```python
from build123d import *

# Parameters (mm, degrees)
BOSS_EXTRUDE1_DEPTH = 5.18
CUT_EXTRUDE4_REACH  = 45.046
SKETCH2_W           = 3.45
SKETCH2_H           = 5.15
CUT_EXTRUDE3_REACH  = 42.402
SKETCH7_R           = 1.575
SKETCH3_W           = 10.5
SKETCH3_H           = 30
SKETCH3_R           = 1.575
BOSS_EXTRUDE2_DEPTH = 1.5


with BuildPart() as part:
    # Sketch1 → Boss-Extrude1 (new body)
    with BuildSketch(Plane(origin=(0, 0, 0), x_dir=(0, 0, -1), z_dir=(1, 0, 0))):
        with BuildLine():
            Line((-5.5, -10.303333333), (-5.5, -17.953333333))
            Line((-5.5, -17.953333333), (3.25, -17.953333333))
            Line((3.25, -17.953333333), (3.25, -19.295))
            Line((3.25, -19.295), (1.25, -19.295))
            Line((1.25, -19.295), (1.25, -19.12))
            Line((1.25, -19.12), (-2.25, -19.12))
            Line((-2.25, -19.12), (-2.25, -19.295))
            Line((-2.25, -19.295), (-4.25, -19.295))
            Line((-4.25, -19.295), (-4.25, -19.12))
            Line((-4.25, -19.12), (-5.5, -19.12))
            Line((-5.5, -19.12), (-5.5, -23.37))
            Line((-5.5, -23.37), (-4.25, -23.37))
            Line((-4.25, -23.37), (-4.25, -23.195))
            Line((-4.25, -23.195), (-2.25, -23.195))
            Line((-2.25, -23.195), (-2.25, -23.37))
            Line((-2.25, -23.37), (1.25, -23.37))
            Line((1.25, -23.37), (1.25, -23.195))
            Line((1.25, -23.195), (3.25, -23.195))
            Line((3.25, -23.195), (3.25, -23.59))
            Line((3.25, -23.59), (-5.5, -23.59))
            Line((-5.5, -23.59), (-5.5, -28.59))
            Line((-5.5, -28.59), (5.72, -28.59))
            Line((5.72, -28.59), (5.72, -14.303333333))
            ThreePointArc((5.72, -14.303333333), (6.012893219, -13.596226552), (6.72, -13.303333333))
            Line((6.72, -13.303333333), (7.061666667, -13.303333333))
            Line((7.061666667, -13.303333333), (7.061666667, -15.303333333))
            Line((7.061666667, -15.303333333), (6.886666667, -15.303333333))
            Line((6.886666667, -15.303333333), (6.886666667, -25.34))
            Line((6.886666667, -25.34), (7.061666667, -25.34))
            Line((7.061666667, -25.34), (7.061666667, -27.34))
            Line((7.061666667, -27.34), (6.886666667, -27.34))
            Line((6.886666667, -27.34), (6.886666667, -28.59))
            Line((6.886666667, -28.59), (11.136666667, -28.59))
            Line((11.136666667, -28.59), (11.136666667, -27.34))
            Line((11.136666667, -27.34), (10.961666667, -27.34))
            Line((10.961666667, -27.34), (10.961666667, -25.34))
            Line((10.961666667, -25.34), (11.136666667, -25.34))
            Line((11.136666667, -25.34), (11.136666667, -15.303333333))
            Line((11.136666667, -15.303333333), (10.961666667, -15.303333333))
            Line((10.961666667, -15.303333333), (10.961666667, -13.303333333))
            Line((10.961666667, -13.303333333), (11.303333333, -13.303333333))
            ThreePointArc((11.303333333, -13.303333333), (12.010440115, -13.596226552), (12.303333333, -14.303333333))
            Line((12.303333333, -14.303333333), (12.303333333, -28.81))
            Line((12.303333333, -28.81), (-5.5, -28.81))
            Line((-5.5, -28.81), (-7, -30.31))
            Line((-7, -30.31), (-7, -36.14))
            Line((-7, -36.14), (-3, -36.14))
            Line((-3, -36.14), (-3, -34.64))
            Line((-3, -34.64), (-5.5, -34.64))
            Line((-5.5, -34.64), (-5.5, -31.31))
            Line((-5.5, -31.31), (17.303333333, -31.31))
            Line((17.303333333, -31.31), (13.803333333, -11.31))
            Line((13.803333333, -11.31), (13.803333333, 0))
            Line((13.803333333, 0), (0, 0))
            Line((0, 0), (0, -2))
            Line((0, -2), (12.303333333, -2))
            Line((12.303333333, -2), (12.303333333, -10.303333333))
            ThreePointArc((12.303333333, -10.303333333), (12.010440115, -11.010440115), (11.303333333, -11.303333333))
            Line((11.303333333, -11.303333333), (10.961666667, -11.303333333))
            Line((10.961666667, -11.303333333), (10.961666667, -9.303333333))
            Line((10.961666667, -9.303333333), (11.136666667, -9.303333333))
            Line((11.136666667, -9.303333333), (11.136666667, -5.47))
            Line((11.136666667, -5.47), (10.961666667, -5.47))
            Line((10.961666667, -5.47), (10.961666667, -3.47))
            Line((10.961666667, -3.47), (11.136666667, -3.47))
            Line((11.136666667, -3.47), (11.136666667, -2.22))
            Line((11.136666667, -2.22), (6.886666667, -2.22))
            Line((6.886666667, -2.22), (6.886666667, -3.47))
            Line((6.886666667, -3.47), (7.061666667, -3.47))
            Line((7.061666667, -3.47), (7.061666667, -5.47))
            Line((7.061666667, -5.47), (6.886666667, -5.47))
            Line((6.886666667, -5.47), (6.886666667, -9.303333333))
            Line((6.886666667, -9.303333333), (7.061666667, -9.303333333))
            Line((7.061666667, -9.303333333), (7.061666667, -11.303333333))
            Line((7.061666667, -11.303333333), (6.72, -11.303333333))
            ThreePointArc((6.72, -11.303333333), (6.012893219, -11.010440115), (5.72, -10.303333333))
            Line((5.72, -10.303333333), (5.72, -2.22))
            Line((5.72, -2.22), (-3, -2.22))
            Line((-3, -2.22), (-3, -6.136666667))
            Line((-3, -6.136666667), (-1.75, -6.136666667))
            Line((-1.75, -6.136666667), (-1.75, -5.961666667))
            Line((-1.75, -5.961666667), (0.25, -5.961666667))
            Line((0.25, -5.961666667), (0.25, -6.136666667))
            Line((0.25, -6.136666667), (1.25, -6.136666667))
            Line((1.25, -6.136666667), (1.25, -5.961666667))
            Line((1.25, -5.961666667), (3.25, -5.961666667))
            Line((3.25, -5.961666667), (3.25, -8.211666667))
            Line((3.25, -8.211666667), (1.25, -8.211666667))
            Line((1.25, -8.211666667), (1.25, -7.886666667))
            Line((1.25, -7.886666667), (0.25, -7.886666667))
            Line((0.25, -7.886666667), (0.25, -8.211666667))
            Line((0.25, -8.211666667), (-1.75, -8.211666667))
            Line((-1.75, -8.211666667), (-1.75, -7.886666667))
            Line((-1.75, -7.886666667), (-3, -7.886666667))
            Line((-3, -7.886666667), (-3, -10.303333333))
            Line((-3, -10.303333333), (-5.5, -10.303333333))
        make_face()
        Polygon((-1.75, -10.303333333), (4.5, -10.303333333), (4.5, -20.37), (3.25, -20.37), (3.25, -20.195), (1.25, -20.195), (1.25, -20.37), (-2.25, -20.37), (-2.25, -20.195), (-4.25, -20.195), (-4.25, -22.295), (-2.25, -22.295), (-2.25, -22.12), (1.25, -22.12), (1.25, -22.295), (3.25, -22.295), (3.25, -22.12), (4.5, -22.12), (4.5, -23.59), (4.72, -23.59), (4.72, -3.72), (-1.75, -3.72), (-1.75, -5.061666667), (0.25, -5.061666667), (0.25, -4.886666667), (1.25, -4.886666667), (1.25, -5.061666667), (3.25, -5.061666667), (3.25, -4.886666667), (4.5, -4.886666667), (4.5, -9.136666667), (3.25, -9.136666667), (3.25, -8.961666667), (1.25, -8.961666667), (1.25, -9.136666667), (0.25, -9.136666667), (0.25, -8.961666667), (-1.75, -8.961666667), align=None, mode=Mode.SUBTRACT)
        Polygon((10.061666667, -27.34), (7.961666667, -27.34), (7.961666667, -25.34), (8.136666667, -25.34), (8.136666667, -15.303333333), (7.961666667, -15.303333333), (7.961666667, -13.303333333), (8.136666667, -13.303333333), (8.136666667, -11.303333333), (7.961666667, -11.303333333), (7.961666667, -9.303333333), (8.136666667, -9.303333333), (8.136666667, -5.47), (7.961666667, -5.47), (7.961666667, -3.47), (10.061666667, -3.47), (10.061666667, -5.47), (9.886666667, -5.47), (9.886666667, -9.303333333), (10.061666667, -9.303333333), (10.061666667, -11.303333333), (9.886666667, -11.303333333), (9.886666667, -13.303333333), (10.061666667, -13.303333333), (10.061666667, -15.303333333), (9.886666667, -15.303333333), (9.886666667, -25.34), (10.061666667, -25.34), align=None, mode=Mode.SUBTRACT)
    extrude(amount=BOSS_EXTRUDE1_DEPTH)

    # Sketch2 → Cut-Extrude4 (cut, up to next)
    with BuildSketch(Plane.XY.offset(5.5), mode=Mode.PRIVATE) as cut_extrude4_sk1:
        with Locations((3.455, -14.128333333)):
            Rectangle(SKETCH2_W, SKETCH2_H)
    cut_extrude4_tool1 = extrude(cut_extrude4_sk1.sketch, amount=-CUT_EXTRUDE4_REACH, mode=Mode.PRIVATE) & part.part
    add(cut_extrude4_tool1.solids().sort_by_distance((3.455, -14.128333, 5.5))[0], mode=Mode.SUBTRACT)

    # Sketch7 → Cut-Extrude3 (cut, up to next)
    with BuildSketch(Plane.ZY, mode=Mode.PRIVATE) as cut_extrude3_sk1:
        with Locations((3, -14.178333333)):
            Circle(SKETCH7_R)
    cut_extrude3_tool1 = extrude(cut_extrude3_sk1.sketch, amount=-CUT_EXTRUDE3_REACH, mode=Mode.PRIVATE) & part.part
    # Sketch7 → Cut-Extrude3 (cut, up to next)
    with BuildSketch(Plane.ZY, mode=Mode.PRIVATE) as cut_extrude3_sk2:
        with Locations((-2, -14.178333333)):
            Circle(SKETCH7_R)
    cut_extrude3_tool2 = extrude(cut_extrude3_sk2.sketch, amount=-CUT_EXTRUDE3_REACH, mode=Mode.PRIVATE) & part.part
    add(cut_extrude3_tool1.solids().sort_by_distance((0, -14.178333, 3))[0], mode=Mode.SUBTRACT)
    add(cut_extrude3_tool2.solids().sort_by_distance((0, -14.178333, -2))[0], mode=Mode.SUBTRACT)

    # Sketch3 → Boss-Extrude2 (add)
    with BuildSketch(Plane.XZ.offset(31.31)):
        with Locations((5.25, -9.5)):
            Rectangle(SKETCH3_W, SKETCH3_H)
        with Locations(Location((7.62, -9.73, 0), (0, 0, 270))):
            Circle(SKETCH3_R, mode=Mode.SUBTRACT)
        with Locations(Location((7.62, -21.73, 0), (0, 0, 270))):
            Circle(SKETCH3_R, mode=Mode.SUBTRACT)
    extrude(amount=-BOSS_EXTRUDE2_DEPTH)


solid = part.part
```
Can you work these out from the model? Positions are in its coordinate system, mm. Round coordinates to 2 decimals unless told otherwise and drop trailing zeros. Loops run counter-clockwise (first coordinate to the right, second up) from the corner with the lowest first, then second, coordinate; pieces in that order, holes last. Notation, with made-up numbers: M 16.25,7.25 L 30.25,7.25 A23 ccw 30.25,23.25 Z; hole C 7,37.5 d3. An arc over 180 degrees is marked long. Write item = value, one per line. Start each with the question number.
(1) Suppose I cut it at D-D on z = -2. Give the number of separate pieces and of enclosed holes in the cut face, plus the area to 3 significant figures.
(2) Suppose I cut it at C-C on z = -7.5. Write out the boundary of the cut face in (x, y).
(3) If we mould it in two halves opening along Z, with no side actions, what happens to faces 1 (the face through (3, -23.37, 1)), 2 (the face through (1, -14, 5.5)), 3 (the face through (3, -7, -4.5)), 4 (the face through (3, -10, -10.962))? For each: released by +Z, released by -Z, zero draft, split by the parting line, or undercut.
(4) Suppose I cut it at B-B on x = 7.62. Write out the boundary of the cut face in (y, z) (3 decimals).
(5) I need wall thicknesses on line 1 along Y through (x, z) = (4.75, -7.5); line 2 along Y through (x, z) = (3.75, -8.5); line 3 along Z through (x, y) = (0.5, -28). Which ranges of each line are inside material? Lowest first, please.
(6) Suppose I cut it at A-A on z = -21.73. Write out the boundary of the cut face in (x, y) (3 decimals).
(7) I'm going to push flat-ended pins straight in: P1, Ø2, axis at x = 5.5, z = 1.5, coming from the +Y side; P2, Ø2.5, axis at x = 2.5, y = -18.5, coming from the +Z side; P3, Ø2, axis at x = 4.5, y = -26.5, coming from the -Z side. Where does each tip first touch, or does it pass through?
Answer block:
q1.separate_pieces = 10
q1.enclosed_holes = 0
q1.area = 99.2 mm²
q2.outline = M 0,-31.31 L 10.5,-31.31 L 10.5,-29.81 L 5.18,-29.81 L 5.18,-28.81 L 0,-28.81 Z; M 0,-28.59 L 5.18,-28.59 L 5.18,-2.22 L 0,-2.22 Z; M 0,-2 L 5.18,-2 L 5.18,0 L 0,0 Z
q3.face_1 = zero draft
q3.face_2 = released by +Z
q3.face_3 = undercut
q3.face_4 = undercut
q4.outline = M -31.31,-24.5 L -29.81,-24.5 L -29.81,-23.305 L -31.31,-23.305 Z; M -31.31,-20.155 L -29.81,-20.155 L -29.81,-11.305 L -31.31,-11.305 Z; M -31.31,-8.155 L -29.81,-8.155 L -29.81,5.5 L -31.31,5.5 Z
q5.line_1 = -31.31 to -28.81, -28.59 to -2.22, -2 to 0
q5.line_2 = -31.31 to -28.81, -28.59 to -27.34, -3.47 to -2.22, -2 to 0
q5.line_3 = -16.72 to -12.3, -11.14 to -6.89, -5.72 to 5.5
q6.outline = M 0,-31.31 L 6.045,-31.31 L 6.045,-29.81 L 0,-29.81 Z; M 9.195,-31.31 L 10.5,-31.31 L 10.5,-29.81 L 9.195,-29.81 Z
q7.P1 = -2.22
q7.P2 = 5.5
q7.P3 = -16.64
